Could you check a few things on this model? Use its own coordinates, in mm. Face numbers are marked on the shaded views. A direction names the side the tool comes from. Give positions to 0.01 mm unless a question says otherwise; leave off trailing zeros. Loops run counter-clockwise (first coordinate to the right, second up) from the corner with the lowest first, then second, coordinate; pieces in that order, holes last. Notation, with made-up numbers: (-26.75, -7) - (-17.75, -7) arc R18 ccw to (-17.75, -3) - close; hole circle Ø7 at (39, 67). An arc over 180 degrees is marked (long way). Write each question's results on one line, items separated by ' | '. Start each with the question number.
Autodesk Inventor part; units mm, degrees
ref_plane "YZ Plane" through (0, 0, 0) normal (1, 0, 0) x (0, 1, 0)
ref_plane "XZ Plane" through (0, 0, 0) normal (0, 1, 0) x (-1, 0, 0)
ref_plane "XY Plane" through (0, 0, 0) normal (0, 0, 1) x (1, 0, 0)
sketch "Sketch1" plane through (0, 0, 0) normal (0, 0, 1) x (1, 0, 0)
  line L0 (42.5, -5) -> (47.4999, -5)
  line L1 (42.5, -10) -> (-42.5, -10)
  line L2 (42.5, -10) -> (42.5, -5)
  line L3 (-42.5, -10) -> (-42.5, -4.9999)
  line L4 (-42.5, -4.9999) -> (-47.5001, -5)
  line L5 (-42.5001, 10) -> (-22.5001, 10)
  line L6 (-42.5001, 10) -> (-42.5001, 5)
  line L7 (42.4999, 10) -> (42.4999, 5)
  line L8 (-42.5001, 5) -> (-47.5001, 5)
  line L9 (42.4999, 5) -> (47.4999, 5)
  line L10 (22.4999, 10) -> (42.4999, 10)
  line L11 (-22.5001, 5) -> (-22.5001, 10)
  line L12 (-22.5001, 5) -> (22.4999, 5)
  line L13 (22.4999, 5) -> (22.4999, 10)
  circle A0 centre (30, 0) radius 2
  circle A1 centre (-30, 0) radius 2
  line L14 (-47.5001, -5) -> (-47.5001, 5)
  line L15 (47.4999, 5) -> (47.4999, -5)
  point P0 (0, 0)
  point P1 (-34.7671, -4.6223)
  dimension "d0" = 4
  dimension "d12" = 30
  dimension "d13" = 4
  dimension "d14" = 30
  dimension "d15" = 20
  dimension "d16" = 20
  dimension "d17" = 42.5
  dimension "d18" = 42.5
  dimension "d21" = 45
  dimension "d32" = 5
  dimension "d33" = 5
extrude "Leap AP" add sketch "Sketch1" along normal blind 5
sketch "Sketch2" plane through (-22.5001, 5, 0) normal (0, 1, 0) x (1, 0, 0)
  line L0 (-25, -56) -> (-20, -56)
  line L1 (70, -56) -> (65, -56)
  line L2 (-20, -56) -> (-20, -69)
  line L3 (-20, -69) -> (-25, -69)
  line L4 (-25, -69) -> (-25, -72)
  line L5 (65, -56) -> (65, -69)
  line L6 (65, -69) -> (70, -69)
  line L7 (70, -69) -> (70, -72)
  line L8 (65, -77) -> (-20, -77)
  line L9 (0, -5) -> (0, 0)
  arc A0 (-25, -72) -> (-20, -77) centre (-20, -72) ccw
  arc A1 (65, -77) -> (70, -72) centre (65, -72) ccw
  line L10 (0, -5) -> (-25, -5)
  line L11 (45, 0) -> (0, 0)
  line L12 (45, 0) -> (45, -5)
  circle A2 centre (0, -73) radius 2
  circle A3 centre (45, -73) radius 2
  line L13 (-25, -56) -> (-25, -5)
  line L14 (70, -56) -> (70, -5)
  circle A4 centre (0, -11.3502) radius 2
  circle A5 centre (45, -11.3502) radius 2
  line L15 (45, -5) -> (70, -5)
  point P0 (-25, -77)
  point P1 (70, -77)
  point P2 (69.9999, -5)
  point P3 (11.4357, -9.3722)
  dimension "d52" = 13
  dimension "d54" = 8
  dimension "d55" = 5
  dimension "d56" = 5
  dimension "d74" = 4
  dimension "d75" = 4
  dimension "d76" = 4
  dimension "d77" = 4
  dimension "d78" = 25
  dimension "d79" = 25
  dimension "d83" = 51
  dimension "d84" = 4
  dimension "d85" = 4
extrude "Leap Base" add sketch "Sketch2" along normal blind 5
sketch "Sketch3" plane through (-42.5001, 5, 0) normal (-1, 0, 0) x (0, 0, 1)
  line L0 (0, -9.9999) -> (5, -9.9999)
  line L1 (0, -9.9999) -> (0, -15)
  line L2 (0, -15) -> (5, -15)
  line L3 (0, 0) -> (5, 0)
  line L4 (5, -9.9999) -> (5, 0)
  line L5 (5, -15) -> (59, -15)
  line L6 (0, 0) -> (0, 5)
  line L7 (69, 5) -> (69, 13)
  line L8 (69, 5) -> (69, -5)
  arc A0 (59, -15) -> (69, -5) centre (59, -5) ccw
  line L9 (69, 13) -> (58.8965, 13)
  line L10 (58.8965, 13) -> (58.8965, 5)
  line L11 (40.1783, 5) -> (40.1783, 13)
  line L12 (40.1783, 13) -> (30.0747, 13)
  line L13 (30.0747, 13) -> (30.0747, 5)
  line L14 (0, 5) -> (30.0747, 5)
  line L15 (40.1783, 5) -> (58.8965, 5)
  point P0 (69, -15)
  point P1 (8.1162, -2.0146)
  dimension "d72" = 10
  dimension "d86" = 8
extrude "2x Leap Side" add sketch "Sketch3" along normal blind 5
sketch "Sketch4" plane through (42.4999, 5, 0) normal (1, 0, 0) x (0, 0, -1)
  line L0 (0, 5) -> (0, -15)
  line L1 (0, -15) -> (-59, -15)
  arc A0 (-69, -5) -> (-59, -15) centre (-59, -5) ccw
  line L2 (-69, -5) -> (-69, 0)
  line L3 (-69, 0) -> (-72, 0)
  line L4 (-72, 0) -> (-72, 5)
  line L5 (-69, 5) -> (-72, 5)
  line L6 (-69, 5) -> (-69, 13)
  line L7 (-69, 13) -> (-58.8965, 13)
  line L8 (-58.8965, 13) -> (-58.8965, 5)
  line L9 (-30.0747, 5) -> (0, 5)
  line L10 (-40.1783, 5) -> (-58.8965, 5)
  line L11 (-40.1783, 5) -> (-40.1783, 13)
  line L12 (-40.1783, 13) -> (-30.0747, 13)
  line L13 (-30.0747, 13) -> (-30.0747, 5)
extrude "Extrusion4" add sketch "Sketch4" along normal blind 5
sketch "Sketch5" plane through (-47.5001, 10, 0) normal (0, 1, 0) x (1, 0, 0)
  line L0 (5, -58.8965) -> (0, -58.8965)
  line L1 (5, -69) -> (5, -58.8965)
  line L2 (5, -69) -> (0, -69)
  line L3 (0, -69) -> (0, -72)
  arc A0 (0, -72) -> (5, -77) centre (5, -72) ccw
  line L4 (5, -77) -> (90, -77)
  arc A1 (90, -77) -> (95, -72) centre (90, -72) ccw
  circle A2 centre (25, -73) radius 2
  circle A3 centre (70, -73) radius 2
  line L5 (0, 0) -> (95, 0)
  line L6 (0, -30.0747) -> (0, 0)
  line L7 (95, -40.1783) -> (95, -58.8965)
  line L8 (95, -30.0747) -> (95, 0)
  line L9 (0, -40.1783) -> (0, -58.8965)
  line L10 (90, -58.8965) -> (90, -69)
  line L11 (90, -58.8965) -> (95, -58.8965)
  line L12 (5, -30.0747) -> (0, -30.0747)
  line L13 (5, -40.1783) -> (5, -30.0747)
  line L14 (5, -40.1783) -> (0, -40.1783)
  line L15 (90, -40.1783) -> (95, -40.1783)
  line L16 (90, -30.0747) -> (90, -40.1783)
  line L17 (90, -30.0747) -> (95, -30.0747)
  line L18 (90, -69) -> (95, -69)
  line L19 (95, -72) -> (95, -69)
  circle A4 centre (25, -11.3502) radius 2
  circle A5 centre (70, -11.3502) radius 2
  point P0 (31.9525, -5.2817)
extrude "Leap Top Base" add sketch "Sketch5" along normal blind 5
properties part number "Attaching Point" material "Nylon 6/6"
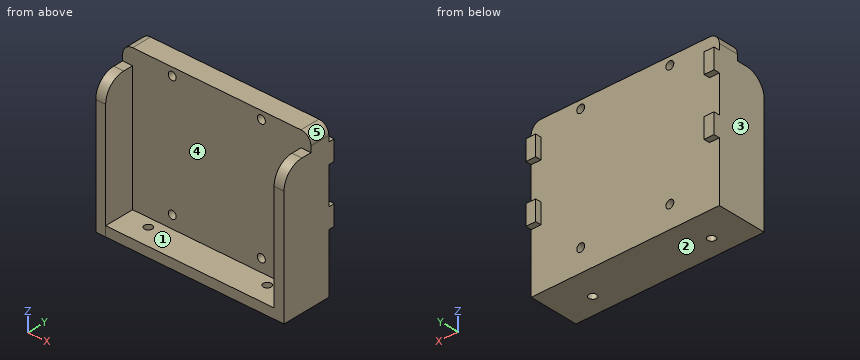
Q1. I want a section at D-D, the plane y = -3.75. List the corners of the cut face in (x, z) for me, then the cut area to 3 significant figures.
Q2. I'm going to push flat-ended pins straight in: pin 1 Ø10 at (x, y) = (-13.5, 1) entering from +Z; pin 2 Ø0.9 at (x, y) = (-45, 17) entering from +Z; pin 3 Ø6 at (x, z) = (-4, 47) entering from -Y; pin 4 Ø3.5 at (x, y) = (45.5, 16) entering from +Z. Where does each tip first touch, or does it pass through?
Q3. I need wall thicknesses on L1, parallel to X at y = 0.25, z = 26; L2, parallel to Y at x = 30, z = 3.1; L3, parallel to Z at x = -14.5, y = 3.75. Which ranges of each line are inside material? Lowest first, please. Write a range as from..to.
Q4. I want a section at B-B, the plane z = 25. List the corners of the cut face in (x, y) for me, then the cut area to 3 significant figures.
Q5. I want a section at C-C, the plane x = 5. List the corners of the cut face in (y, z) for me, then the cut area to 3 significant figures.
Q6. If we mould it in two halves opening along X, with no side actions, what happens to the marked faces 3, 4 and 5? For each: +X half, -X half, draft (parallel to the pull), parting line (faces both ways), or undercut.
Q7. I want a section at A-A, the plane x = -30. List the corners of the cut face in (y, z) for me.
Q8. Which directions (+Z, -Z, +X, -X, +Y, -Y) give clear straight access to the entire face, cutting with the end or side of a thin tool? Please do the marked faces 1 and 2.
Conclusion:
1) outline: (-47.5, 0) - (47.5, 0) - (47.5, 68.27) - (42.5, 68.27) - (42.5, 5) - (-42.5, 5) - (-42.5, 68.27) - (-47.5, 68.27) - close | area: 1,110 mm^2
2) pin 1: z = 77 | pin 2: z = 69 | pin 3: y = 5 | pin 4: z = 76.75
3) L1: -47.5..-42.5, 42.5..47.5 | L2: -10..-2, 2..15 | L3: 0..5
4) outline: (-47.5, -10) - (-42.5, -10) - (-42.5, 5) - (42.5, 5) - (42.5, -10) - (47.5, -10) - (47.5, 15) - (-47.5, 15) - close | area: 1,100 mm^2
5) outline: (-10, 0) - (15, 0) - (15, 77) - (5, 77) - (5, 5) - (-10, 5) - close | area: 845 mm^2
6) face 3: -X half | face 4: undercut | face 5: +X half
7) outline: (-10, 0) - (-2, 0) - (-2, 5) - (-10, 5) - close; (2, 0) - (15, 0) - (15, 77) - (5, 77) - (5, 5) - (2, 5) - close
8) face 1: +Z, -Y | face 2: -Z, +X, -X, +Y, -Y
